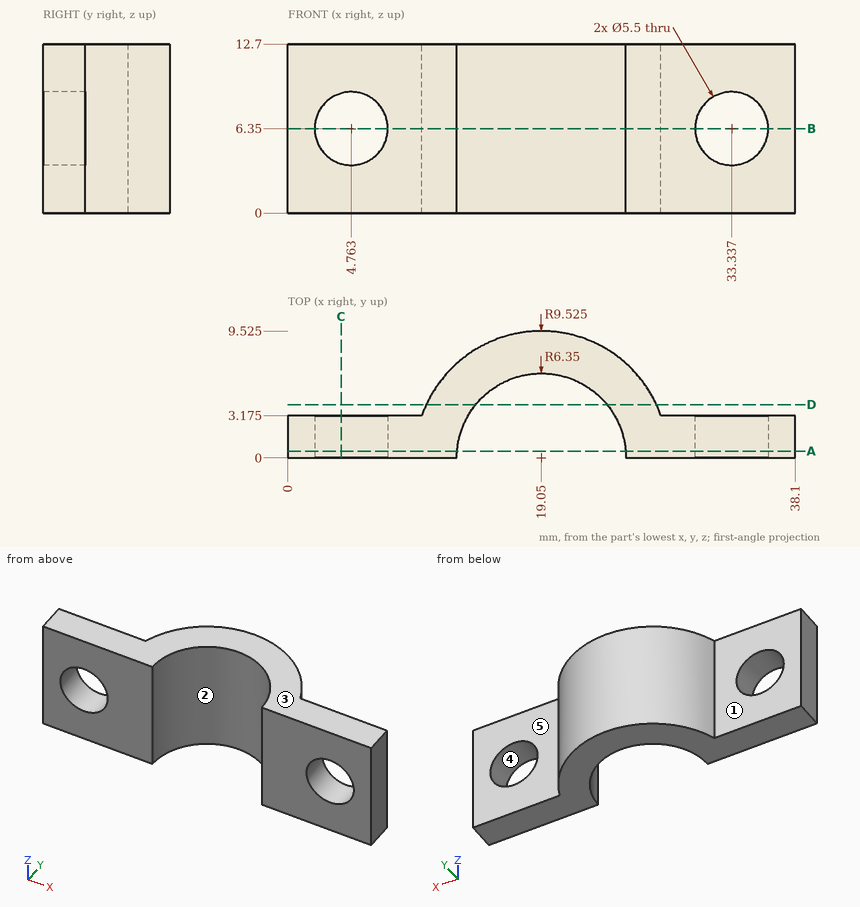
Job drawing, mm, ordinate dimensions from the low corner. One solid piece. A direction names the side the tool comes from. Give positions to 0.01 mm unless a question says otherwise; leave off trailing zeros. Loops run counter-clockwise (first coordinate to the right, second up) from the corner with the lowest first, then second, coordinate; pieces in that order, holes last.
Item 1: Slice it at C-C, the plane x = 4. List the corners of the cut face in (y, z) (1 decimal).
Answers follow:
outline: (0, 0) - (3.2, 0) - (3.2, 3.7) - (0, 3.7) - close; (0, 9) - (3.2, 9) - (3.2, 12.7) - (0, 12.7) - close
Item 2: Drill centre lines: line 1 (Y direction, x = 31, z = 2) (1 decimal); line 2 (X direction, y = 4, z = 2.5) (1 decimal); line 3 (Y direction, x = 26.5, z = 2.5) (1 decimal). Where is each one in solid material? Low to high.
Answers follow:
line 1: y = 0 to 3.2
line 2: x = 10.4 to 14.1, 24 to 27.7
line 3: y = 0 to 5.9
Item 3: Which spindle directions (+Z, -Z, +X, -X, +Y, -Y) get a long thin tool onto all of the face, cutting with end or side? Do the marked faces 1 and 2. Say none if no direction does.
Answers follow:
face 1: +Z, -Z, -X, +Y
face 2: +Z, -Z, -Y
Item 4: Slice it at D-D, the plane y = 4. List the corners of the cut face in (x, z) (1 decimal).
Answers follow:
outline: (10.4, 0) - (14.1, 0) - (14.1, 12.7) - (10.4, 12.7) - close; (24, 0) - (27.7, 0) - (27.7, 12.7) - (24, 12.7) - close
Item 5: Slice it at A-A, the plane y = 0.5. List the corners of the cut face in (x, z).
Answers follow:
outline: (0, 0) - (12.72, 0) - (12.72, 12.7) - (0, 12.7) - close; (25.38, 0) - (38.1, 0) - (38.1, 12.7) - (25.38, 12.7) - close; hole circle Ø5.5 at (4.76, 6.35); hole circle Ø5.5 at (33.34, 6.35)
Item 6: Slice it at B-B, the plane z = 6.35. Give the number of separate pieces and of enclosed holes in the cut face, and give its area (3 significant figures).
Answers follow:
separate pieces: 3
enclosed holes: 0
area: 106 mm2
Item 7: Pull direction Z, two halves, no side cores. Call the marked faces 3, 4 and 5: released by +Z, released by -Z, zero draft, split by the parting line, or undercut.
Answers follow:
face 3: released by +Z
face 4: undercut
face 5: zero draft
Item 8: Flat gauge pins, fed straight in: pin 1 (3 mm diameter, centred on x = 6.5, z = 4.5, fed in from +Y) (1 decimal); pin 2 (2 mm diameter, centred on y = 5, z = 10.5, fed in from +X) (1 decimal); pin 3 (3 mm diameter, centred on x = 6, y = 5, fed in from +Z) (3 decimals); pin 4 (5 mm diameter, centred on y = 4.5, z = 9, fed in from +X). Where does each tip first touch, or does it go through?
Answers follow:
pin 1: stops at y = 3.2
pin 2: stops at x = 27.7
pin 3: passes through
pin 4: stops at x = 38.1
